Design review of the part shown in the three views and the two pictorial views. Dimensions are in mm from the part's minimum x, y and z. Give positions to 0.01 mm unless a question says otherwise; leave off trailing zeros. Write each loop counter-clockwise with the first axis right and the second up, starting at its lowest first coordinate (ties: lowest second). Pieces come first, ordered by that corner, then holes. Notation, with made-up numbers: (-40, 85) -> (-14, 85) arc R24 cw to (-14, 108) -> close; hole circle Ø6 at (-40, -28.75). An arc over 180 degrees is marked (long way). Return JSON: item names as keys, results as strings. Group by question number.
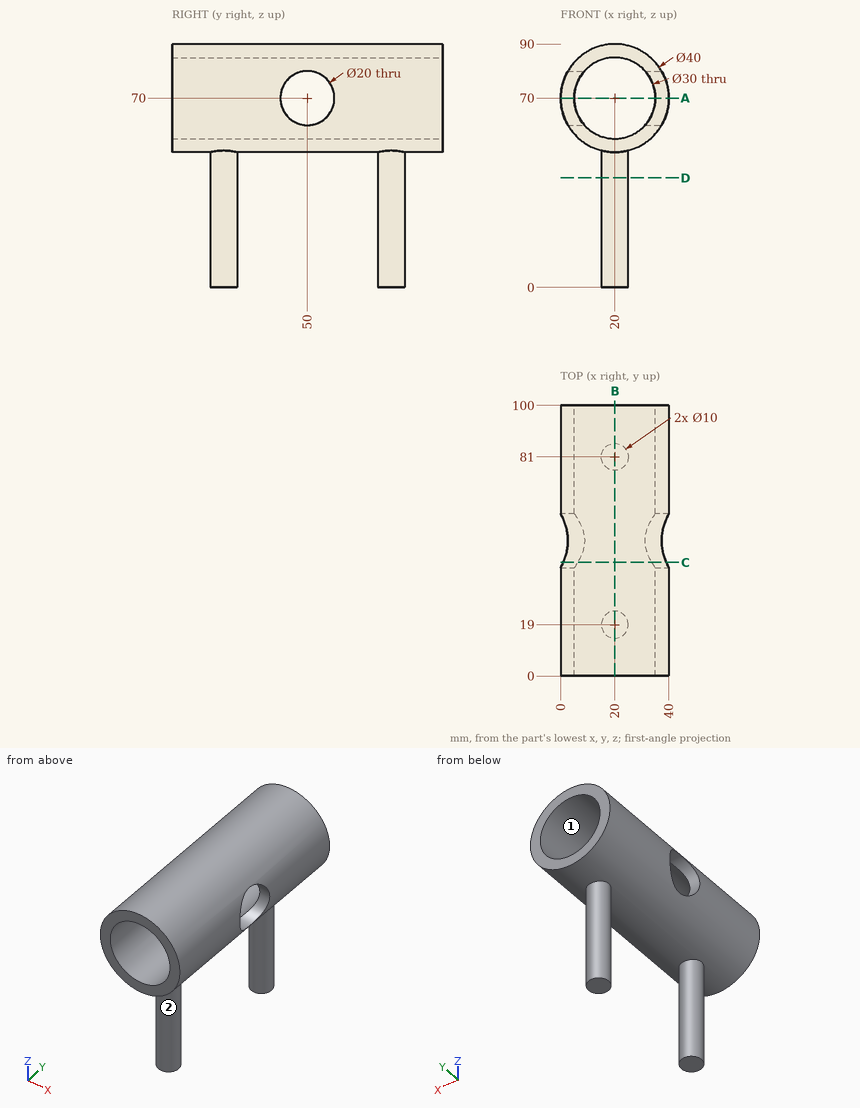
Q1. For L1, parallel to Z at x = 20, y = 35; L2, parallel to Z at x = 18.5, y = 83; L3, parallel to Y at x = 35, z = 67, list the stretches that pass through material, from the lowest coordinate up. Write a range as from..to.
Q2. Insertion check: pin 1 (6 mm diameter, centred on x = 23, y = 60.5, fed in from -Z); pin 2 (2 mm diameter, centred on x = 7.5, y = 57.5, fed in from -Z); pin 3 (8 mm diameter, centred on x = 10.5, y = 56, fed in from -Z). Each pin has a flat end and moves straight along its axis. Give the tip position at first contact, or say it passes through.
Q3. Take a section at D-D, the plane z = 40.5. Give the boundary of the cut face in (x, y), plus the area to 3 significant figures.
Q4. Take a section at A-A, the plane z = 70. Give the boundary of the cut face in (x, y).
Q5. Take a section at C-C, the plane y = 42. Give the boundary of the cut face in (x, z), plus the area to 3 significant figures.
Q6. Mouldability with a two-part tool opening along X and no side actions: class the marked faces 1 and 2 as +X half, -X half, draft (parallel to the pull), parting line (faces both ways), or undercut.
Q7. Take a section at B-B, the plane x = 20. Give the boundary of the cut face in (y, z).
Final values:
{
 "1": {"L1": "z = 50..55, 85..90", "L2": "z = 0..55.08, 84.92..89.94", "L3": "y = 0..40.46, 59.54..100"},
 "2": {"pin 1": "stops at z = 50", "pin 2": "stops at z = 53.64", "pin 3": "stops at z = 50.77"},
 "3": {"outline": "circle Ø10 at (20, 19); circle Ø10 at (20, 81)", "area": "157 mm²"},
 "4": {"outline": "(0, 0) -> (5, 0) -> (5, 40) -> (0, 40) -> close; (0, 60) -> (5, 60) -> (5, 100) -> (0, 100) -> close; (35, 0) -> (40, 0) -> (40, 40) -> (35, 40) -> close; (35, 60) -> (40, 60) -> (40, 100) -> (35, 100) -> close"},
 "5": {"outline": "(0.92, 64) arc R20 ccw to (39.08, 64) -> (33.75, 64) arc R15 cw to (6.25, 64) -> close; (0.92, 76) -> (6.25, 76) arc R15 cw to (33.75, 76) -> (39.08, 76) arc R20 ccw to start", "area": "427 mm²"},
 "6": {"face 1": "undercut", "face 2": "parting line"},
 "7": {"outline": "(0, 50) -> (14, 50) -> (14, 0) -> (24, 0) -> (24, 50) -> (76, 50) -> (76, 0) -> (86, 0) -> (86, 50) -> (100, 50) -> (100, 55) -> (0, 55) -> close; (0, 85) -> (100, 85) -> (100, 90) -> (0, 90) -> close"}
}
